Verification items for this drawing (mm, ordinates from the low corner). Round coordinates to 2 decimals unless told otherwise and drop trailing zeros. Order: outer loops, then holes, each group sorted by start corner. A loop starts at its lowest first (then second) coordinate and runs counter-clockwise, first axis right, second up. Notation, with made-up numbers: M 41,20.5 L 63,20.5 A34 cw 63,59.5 Z; hole C 46,-32 d3. An arc over 180 degrees is marked long. Return JSON: item names as keys, results as strings. Group by question number.
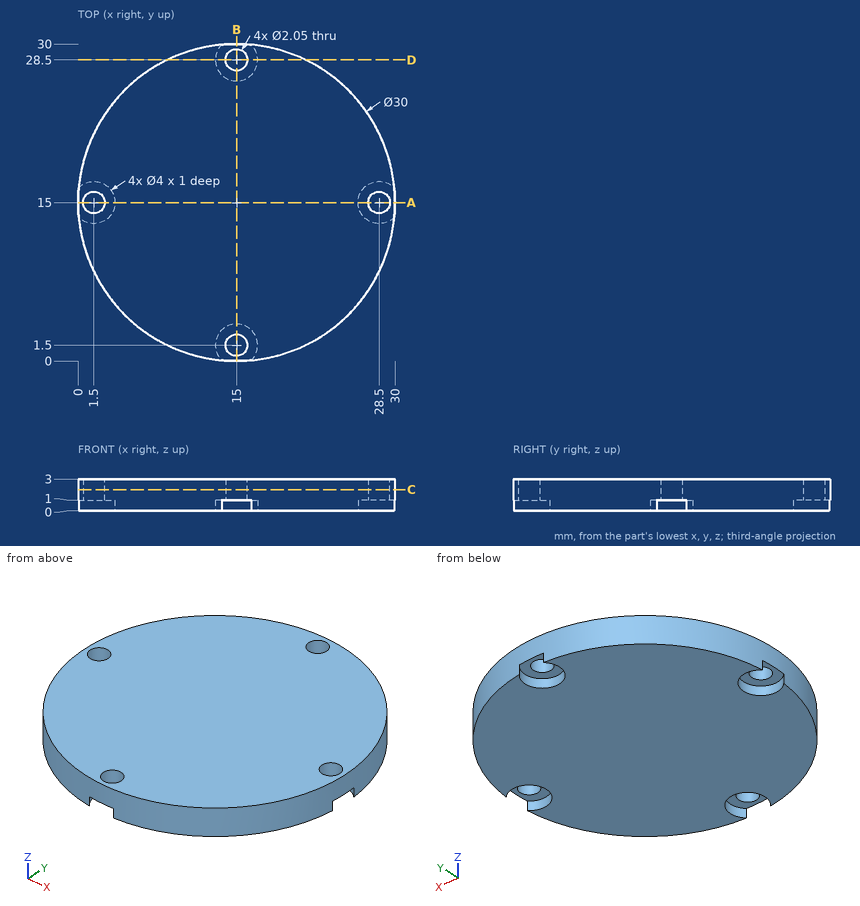
Q1. Section check C-C on z = 2. Record the cut outline in (x, y) (3 decimals), plus the area to 3 significant figures.
Q2. Depth check by flat-ended pin: pin 1 Ø3.5 at (x, y) = (15, 1.5) entering from -Z; pin 2 Ø5 at (x, y) = (1.5, 15) entering from -Z; pin 3 Ø1 at (y, z) = (18.5, 0.5) entering from -X; pin 4 Ø1 at (x, z) = (4, 0.5) entering from -Y. Enter the tip coordinate at first touch or a pass-through.
Q3. Section check D-D on y = 28.5. Record the cut outline in (x, z) (3 decimals), plus the area to 3 significant figures.
Q4. Material ranges on line 1 along X through (y, z) = (15, 2.45) (3 decimals); line 2 along X through (y, z) = (15, 0.7), recorded low to high.
Q5. Section check A-A on y = 15. Record the cut outline in (x, z) (3 decimals), plus the area to 3 significant figures.
Geometry check:
{
 "1": {"outline": "C 15,15 d30; hole C 1.5,15 d2.05; hole C 15,1.5 d2.05; hole C 15,28.5 d2.05; hole C 28.5,15 d2.05", "area": "694 mm^2"},
 "2": {"pin 1": "stops at z = 1", "pin 2": "stops at z = 0", "pin 3": "stops at x = 0.3", "pin 4": "stops at y = 4.29"},
 "3": {"outline": "M 8.462,0 L 13,0 L 13,1 L 13.975,1 L 13.975,3 L 8.462,3 Z; M 16.025,1 L 17,1 L 17,0 L 21.538,0 L 21.538,3 L 16.025,3 Z", "area": "31.1 mm^2"},
 "4": {"line 1": "x = 0 to 0.475, 2.525 to 27.475, 29.525 to 30", "line 2": "x = 3.5 to 26.5"},
 "5": {"outline": "M 0,1 L 0.475,1 L 0.475,3 L 0,3 Z; M 2.525,1 L 3.5,1 L 3.5,0 L 26.5,0 L 26.5,1 L 27.475,1 L 27.475,3 L 2.525,3 Z; M 29.525,1 L 30,1 L 30,3 L 29.525,3 Z", "area": "74.8 mm^2"}
}
